```python
from build123d import *

# Parameters (mm, degrees)
BOSS_EXTRUDE2_DEPTH = 12.25
FILLET1_RADIUS      = 6.125
FILLET1_LENGTH      = 1
FILLET3_R           = 1


with BuildPart() as part:
    # Sketch1 → Boss-Extrude2 (new body)
    with BuildSketch(Plane.XY):
        Polygon((0, 0), (-17.3, 0), (-17.3, 11), (0, 11), (0, 10), (-16.3, 10), (-16.3, 1), (0, 1), align=None)
    extrude(amount=BOSS_EXTRUDE2_DEPTH)

    # Fillet1: full round fillet: the end face becomes a half cylinder, R = half its width
    fillet1_face = Plane((0, 10.5, 6.125), x_dir=(0, -1, 0), z_dir=(1, 0, 0))  # on the end face: x along it, z out of the body
    fillet1_slab = fillet1_face.offset(-FILLET1_RADIUS / 2) * Box(FILLET1_LENGTH, 2 * FILLET1_RADIUS, FILLET1_RADIUS, mode=Mode.PRIVATE)  # the body's end, R deep
    fillet1_round = Plane((-6.125, 10.5, 6.125), x_dir=(1, 0, 0), z_dir=(0, -1, 0)) * Cylinder(FILLET1_RADIUS, FILLET1_LENGTH, mode=Mode.PRIVATE)  # its axis R under the face
    add(fillet1_slab - fillet1_round, mode=Mode.SUBTRACT)

    # Fillet3
    fillet3_edges = [part.edges().sort_by_distance(p)[0] for p in [
        (0, 0.5, 0),
        (-17.3, 0, 6.125),
        (-17.3, 11, 6.125),
        (-16.3, 10, 6.125),
        (-16.3, 1, 6.125),
        (0, 0.5, 12.25),
    ]]
    fillet(fillet3_edges, radius=FILLET3_R)


solid = part.part
```
Here's how the part is built. I have some questions about the finished solid (model axes, mm). A direction names the side the tool comes from. Give positions to 0.01 mm unless a question says otherwise; leave off trailing zeros. Order: outer loops, then holes, each group sorted by start corner. A loop starts at its lowest first (then second) coordinate and runs counter-clockwise, first axis right, second up. Notation, with made-up numbers: M 53.25,69 L 71.25,69 A17 ccw 71.25,88 Z; hole C 45,80 d5. An arc over 180 degrees is marked long. Use a Markdown table: item, result. Add a question column.
1. Suppose I cut it at A-A (x = -10). List the corners of the cut face in (y, z) for me.
2. I need wall thicknesses on probe 1 along Y at (x, z) = (-5.75, 10.5); probe 2 along X at (y, z) = (5.25, 1.5); probe 3 along Y at (x, z) = (-16, 0.75). Which ranges of each line are inside material? Lowest first, please. Write a range as from..to.
3. If we mould it in two halves opening along Y, with no side actions, what happens to faces 4 (the flat face through (-8, 0, 6)), 5 (the flat face through (-8, 1, 6)), 6 (the flat face through (0, 0.5, 6.1)), 7 (the cylindrical face through (-16.999, 10.715, 6.211))? For each: +Y half, -Y half, draft (parallel to the pull), parting line (faces both ways), or undercut.
4. On a 3-axis mill with a long thin cutter (end or side, diameter ignored), from which of +Z, -Z, +X, -X, +Y, -Y can I reach the whole of each face in a straight line? I mean faces 1 (the cylindrical face through (-15.999, 9.715, 6.211)), 2 (the cylindrical face through (-16.999, 0.285, 6.211)), 3 (the cylindrical face through (0, 10.5, 6)). Say none if no direction works.
5. Suppose I cut it at D-D (x = -1.25). List the corners of the cut face in (y, z) for me, and give its area (3 significant figures).
6. Suppose I cut it at C-C (y = 7). List the corners of the cut face in (x, z) for me.
7. Suppose I cut it at B-B (z = 2). List the corners of the cut face in (x, y) for me.
8. For pin 1 Ø3.5 at (y, z) = (6.5, 8) entering from +X, with a flat end and sliding along its axis, tell me the tip position at first contact or that it passes through.
Results list:
| question | item | result |
|---|---|---|
| 1 | outline | M 0,0 L 1,0 L 1,12.25 L 0,12.25 Z; M 10,0 L 11,0 L 11,12.25 L 10,12.25 Z |
| 2 | probe 1 | y = 0..1, 10..11 |
| 2 | probe 2 | x = -17.3..-16.3 |
| 2 | probe 3 | y = 0..1.29, 9.71..11 |
| 3 | face 4 | -Y half |
| 3 | face 5 | undercut |
| 3 | face 6 | draft |
| 3 | face 7 | +Y half |
| 4 | face 1 | +Z, -Z, +X |
| 4 | face 2 | +Z, -Z, -X, -Y |
| 4 | face 3 | +X, +Y |
| 5 | outline | M 0,0 L 1,0 L 1,12.25 L 0,12.25 Z; M 10,2.42 L 11,2.42 L 11,9.83 L 10,9.83 Z |
| 5 | area | 19.7 mm² |
| 6 | outline | M -17.3,0 L -16.3,0 L -16.3,12.25 L -17.3,12.25 Z |
| 7 | outline | M -17.3,1 A1 ccw -16.3,0 L 0,0 L 0,1 L -15.3,1 A1 cw -16.3,2 L -16.3,9 A1 cw -15.3,10 L -1.6,10 L -1.6,11 L -16.3,11 A1 ccw -17.3,10 Z |
| 8 | pin 1 | stops at x = -16.3 |
